Geometry check sheet. Reference: drawing and pictorial views, mm from the part's lowest x, y, z. Coordinates: 2 decimals unless noted, no trailing zeros. Write each loop counter-clockwise with the first axis right and the second up, starting at its lowest first coordinate (ties: lowest second). Pieces come first, ordered by that corner, then holes. Notation, with made-up numbers: M 48.5,-32.5 L 68.5,-32.5 A34 cw 68.5,5.5 Z; hole C 88.25,-15.75 d9. An arc over 180 degrees is marked long. One line per item, written item: value.
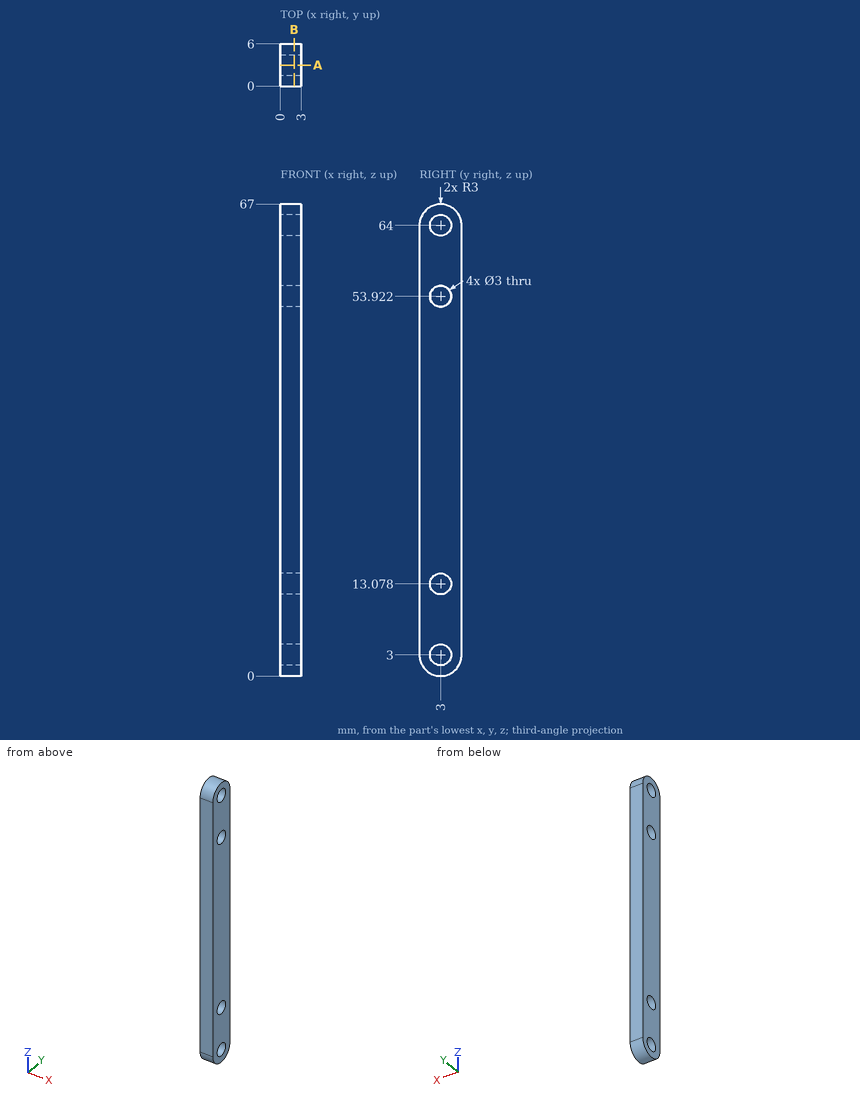
Item 1: Cross-section at B-B, the plane x = 1.95. Enter the section's corners in (y, z), and give its area (3 significant figures).
The answers:
outline: M 0,3 A3 ccw 6,3 L 6,64 A3 ccw 0,64 Z; hole C 3,3 d3; hole C 3,13.08 d3; hole C 3,53.92 d3; hole C 3,64 d3
area: 366 mm²
Item 2: Cross-section at A-A, the plane y = 3. Enter the section's corners in (x, z).
The answers:
outline: M 0,0 L 3,0 L 3,1.5 L 0,1.5 Z; M 0,4.5 L 3,4.5 L 3,11.58 L 0,11.58 Z; M 0,14.58 L 3,14.58 L 3,52.42 L 0,52.42 Z; M 0,55.42 L 3,55.42 L 3,62.5 L 0,62.5 Z; M 0,65.5 L 3,65.5 L 3,67 L 0,67 Z
Item 3: Go/stop test with a flat-tipped pin: P1, Ø3, axis at y = 1, z = 26, coming from the -X side. Record where the tip stops, or that it passes through.
The answers:
P1: stops at x = 0
Item 4: Scan lines: line 1 (Z direction, x = 1.45, y = 3); line 2 (Y direction, x = 1.5, z = 3); line 3 (Z direction, x = 1.25, y = 3.6). Record each from-to range of solid material in increasing order.
The answers:
line 1: z = 0 to 1.5, 4.5 to 11.58, 14.58 to 52.42, 55.42 to 62.5, 65.5 to 67
line 2: y = 0 to 1.5, 4.5 to 6
line 3: z = 0.06 to 1.63, 4.37 to 11.7, 14.45 to 52.55, 55.3 to 62.63, 65.37 to 66.94
